Check sheet for the modelled part. Datum: model origin and axes. Units: mm. A direction names the side the tool comes from. Round coordinates to 2 decimals unless told otherwise and drop trailing zeros. Loops run counter-clockwise (first coordinate to the right, second up) from the corner with the lowest first, then second, coordinate; pieces in that order, holes last. Notation, with made-up numbers: (65.5, 39.25) -> (104.5, 39.25) arc R15 cw to (104.5, 45.25) -> close; hole circle Ø10 at (84.5, 83). An arc over 180 degrees is marked (long way). Use one line per item in the form item = value. Start each with the question number.
(1) Set-up check for faces 1 (the flat face through (0, 2, -21.588)), 2 (the flat face through (0.475, 2, -7)), 3 (the flat face through (-1, 2, 20)): record each of +Z, -Z, +X, -X, +Y, -Y from which the full face is reachable in a straight line by a thin tool's end or side.
(2) Sectioned sample at B-B (y = 1.9). Record the cut outline in (x, z) (1 decimal).
(3) Draft check along Z on faces 4 (the flat face through (0, 3.175, 0)), 5 (the flat face through (1, 2, -5.563)), 6 (the flat face through (0, 2, 18.413)). Enter one of: released by +Z, released by -Z, zero draft, split by the parting line, or undercut.
(4) Material ranges on probe 1 along X at (y, z) = (0.15, 20); probe 2 along Z at (x, y) = (1.5, 2.2); probe 3 along Z at (x, y) = (0.75, 0.2), recorded low to high. Write a range as [from, to].
(5) Sectioned sample at A-A (x = 2). Record the cut outline in (y, z) (1 decimal), and give its area (3 significant figures).
(6) Go/stop test with a flat-tipped pin: pin 1 (1.6 mm diameter, centred on x = 0, y = 1, fed in from +Z). Record where the tip stops, or that it passes through.
(7) Sectioned sample at C-C (x = -0.25). Record the cut outline in (y, z) (1 decimal), and give its area (3 significant figures).
from build123d import *

# Parameters (mm, degrees)
SKETCH1_W           = 2.05
SKETCH1_H           = 2.05
BOSS_EXTRUDE1_DEPTH = 3.175


with BuildPart() as part:
    # Sketch1 → Boss-Extrude1 (new body)
    with BuildSketch(Plane(origin=(0, 0, 0), x_dir=(1, 0, 0), z_dir=(0, 1, 0))):
        Polygon((1, -21.587500005), (3.5, -21.587500005), (3.5, 21.587500005), (-3.5, 21.587500005), (-3.5, -14.587500005), (-3.5, -17.087500005), (-3.5, -19.087500005), (-3.5, -21.587500005), (-1, -21.587500005), (-1, -18.412500005), (1, -18.412500005), align=None)
        with Locations((1.5, 6.587500005)):
            Rectangle(SKETCH1_W, SKETCH1_H, mode=Mode.SUBTRACT)
    extrude(amount=BOSS_EXTRUDE1_DEPTH)


solid = part.part
Checks:
q1.face_1 = -Z, +X, -X, +Y, -Y
q1.face_2 = +Y, -Y
q1.face_3 = +Z, +Y, -Y
q2.outline = (-3.5, -21.6) -> (3.5, -21.6) -> (3.5, 21.6) -> (1, 21.6) -> (1, 18.4) -> (-1, 18.4) -> (-1, 21.6) -> (-3.5, 21.6) -> close; hole (0.5, -7.6) -> (2.5, -7.6) -> (2.5, -5.6) -> (0.5, -5.6) -> close
q3.face_4 = zero draft
q3.face_5 = undercut
q3.face_6 = released by +Z
q4.probe_1 = [-3.5, -1], [1, 3.5]
q4.probe_2 = [-21.59, -7.61], [-5.56, 21.59]
q4.probe_3 = [-21.59, -7.61], [-5.56, 18.41]
q5.outline = (0, -21.6) -> (3.2, -21.6) -> (3.2, -7.6) -> (0, -7.6) -> close; (0, -5.6) -> (3.2, -5.6) -> (3.2, 21.6) -> (0, 21.6) -> close
q5.area = 131 mm2
q6.pin_1 = 18.41
q7.outline = (0, -21.6) -> (3.2, -21.6) -> (3.2, 18.4) -> (0, 18.4) -> close
q7.area = 127 mm2
